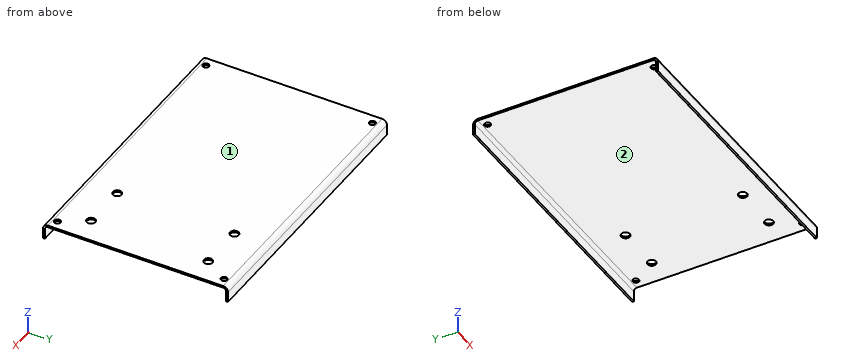
Autodesk Inventor part; units mm, degrees
ref_plane "YZ Plane" through (0, 0, 0) normal (1, 0, 0) x (0, 1, 0)
ref_plane "XZ Plane" through (0, 0, 0) normal (0, 1, 0) x (-1, 0, 0)
ref_plane "XY Plane" through (0, 0, 0) normal (0, 0, 1) x (1, 0, 0)
sketch "Sketch1" plane through (0, 0, 0) normal (0, 0, 1) x (1, 0, 0)
  line L0 (-225, 150) -> (225, 150)
  line L1 (225, 150) -> (225, -150)
  line L2 (225, -150) -> (-225, -150)
  line L3 (-225, -150) -> (-225, 150)
  line L4 (-225, 150) -> (225, -150) construction
  point P0 (0, 0)
  point P1 (0, 0)
  dimension "d0" = 450
  dimension "d1" = 300
extrude "Plate1" add sketch "Sketch1" against normal blind 3
sketch "Sketch2" plane through (0, 0, 0) normal (0, 0, 1) x (1, 0, 0)
  line L0 (111, 95) -> (185, 95) construction
  line L1 (185, 95) -> (185, -95) construction
  line L2 (185, -95) -> (111, -95) construction
  line L3 (111, -95) -> (111, 95) construction
  line L4 (225, -150) -> (225, 150)
  point P0 (0, 0)
  point P1 (111, 0)
  dimension "d3" = 74
  dimension "d4" = 190
  dimension "d5" = 40
hole "Hole1" at (111, 95, 0) at (185, 95, 0) at (111, -95, 0) at (185, -95, 0) direction (0, 0, -1) diameter 14 end through all
sketch "Sketch3" plane through (0, 0, 0) normal (0, 0, 1) x (1, 0, 0)
  line L0 (-210, 135) -> (210, 135) construction
  line L1 (210, 135) -> (210, -135) construction
  line L2 (210, -135) -> (-210, -135) construction
  line L3 (-210, -135) -> (-210, 135) construction
  line L4 (-210, 135) -> (210, -135) construction
  point P0 (0, 0)
  point P1 (0, 0)
  dimension "d14" = 270
  dimension "d15" = 420
hole "Hole2" at (-210, 135, 0) at (210, 135, 0) at (210, -135, 0) at (-210, -135, 0) direction (0, 0, -1) diameter 10 end through all
sketch "Sketch4" plane through (-225, -147, 0) normal (0, -1, 0) x (1, 0, 0)
  line L0 (450, 0) -> (0, 0)
  line L1 (0, 0) -> (0, -25)
  line L2 (0, -25) -> (450, -25)
  line L3 (450, -25) -> (450, 0)
edge flange "Flange1" height 25 angle 90 thickness 3 bend radius 5 thickness toward (0, -1, 0) relief round relief width 3 relief depth 1.5 corner gap 5 corner form 0 edges at (0, -150, -3) (0, 150, -3) wall of the first edge with corners at (225, -147, 0) (-225, -147, 0) (-225, -147, -25) (225, -147, -25)
bend "Bend1"
corner "Corner1"
equation "\"d11\" = Thickness"
equation "\"d2\" = Thickness"
equation "\"d23\" = BendReliefWidth"
equation "\"d24\" = BendReliefDepth"
equation "\"d25\" = MinimumRemnant"
equation "\"d26\" = TransitionRadius"
equation "\"d29\" = BendRadius"
equation "\"d30\" = CornerReliefSize"
equation "\"d31\" = GapSize"
equation "\"d32\" = JacobiRadiusSize"
equation "\"BendReliefWidth\" = Thickness"
equation "\"BendReliefDepth\" = 0.5 * Thickness"
equation "\"CornerReliefSize\" = 4 * Thickness"
equation "\"MinimumRemnant\" = 2 * Thickness"
equation "\"TransitionRadius\" = BendRadius"
equation "\"JacobiRadiusSize\" = BendRadius"
equation "\"GapSize\" = Thickness"
properties part number "Purity pump plate" material "Stainless Steel"
Model file for the job. Use its own axes, mm. Face numbers are marked on the shaded views. Give positions to 0.01 mm unless a question says otherwise; leave off trailing zeros. Loops run counter-clockwise (first coordinate to the right, second up) from the corner with the lowest first, then second, coordinate; pieces in that order, holes last. Notation, with made-up numbers: M 68.5,37 L 105.5,37 A16 ccw 105.5,44 Z; hole C 31.25,-31.5 d4. An arc over 180 degrees is marked long. Use one line per item in the form item = value.
Item 1: Slice it at D-D on x = 111. List the corners of the cut face in (y, z).
Filled in:
outline = M -150,-25 L -147,-25 L -147,-8 A5 cw -142,-3 L -102,-3 L -102,0 L -142,0 A8 ccw -150,-8 Z; M -88,-3 L 88,-3 L 88,0 L -88,0 Z; M 102,-3 L 142,-3 A5 cw 147,-8 L 147,-25 L 150,-25 L 150,-8 A8 ccw 142,0 L 102,0 Z
Item 2: Drill centre lines: L1, parallel to X at y = -135, z = -1.7; L2, parallel to X at y = 95, z = -1.55; L3, parallel to Y at x = -90.5, z = -13.5. Where is each one in solid material? Low to high.
Filled in:
L1 = -225 to -215, -205 to 205, 215 to 225
L2 = -225 to 104, 118 to 178, 192 to 225
L3 = -150 to -147, 147 to 150
Item 3: Flat gauge pin, fed straight in: pin 1 Ø3 at (x, y) = (-25.5, 13) entering from -Z. Where does the tip first touch, or does it go through?
Filled in:
pin_1 = -3
Item 4: Slice it at C-C on y = -135. List the corners of the cut face in (x, z).
Filled in:
outline = M -225,-3 L -215,-3 L -215,0 L -225,0 Z; M -205,-3 L 205,-3 L 205,0 L -205,0 Z; M 215,-3 L 225,-3 L 225,0 L 215,0 Z
Item 5: Slice it at B-B on z = -19. List the corners of the cut face in (x, y), and give its area (3 significant figures).
Filled in:
outline = M -225,-150 L 225,-150 L 225,-147 L -225,-147 Z; M -225,147 L 225,147 L 225,150 L -225,150 Z
area = 2,700 mm^2
Item 6: Slice it at A-A on x = 210. List the corners of the cut face in (y, z), and give its area (3 significant figures).
Filled in:
outline = M -150,-25 L -147,-25 L -147,-8 A5 cw -142,-3 L -140,-3 L -140,0 L -142,0 A8 ccw -150,-8 Z; M -130,-3 L 130,-3 L 130,0 L -130,0 Z; M 140,-3 L 142,-3 A5 cw 147,-8 L 147,-25 L 150,-25 L 150,-8 A8 ccw 142,0 L 140,0 Z
area = 955 mm^2
Item 7: Two-plate mould, pull along Y, no slides. Class the marked faces 1 and 2: released by +Y, released by -Y, zero draft, split by the parting line, or undercut.
Filled in:
face_1 = zero draft
face_2 = undercut
